```python
from build123d import *

# Parameters (mm, degrees)
SKETCH1_R           = 2
BOSS_EXTRUDE1_DEPTH = 8


with BuildPart() as part:
    # Sketch1 → Boss-Extrude1 (new body)
    with BuildSketch(Plane.XY):
        Polygon((-111.736544033, -14.131727984), (-9.968599743, -14.131727984), (0, -14.131727984), (0, 18.131727984), (-10, 18.131727984), (-10, 10.368272016), (-111.736544033, 10.368272016), (-111.736544033, 18.131727984), (-140, 18.131727984), (-140, -14.131727984), align=None)
        with Locations((-134, 8.131727984)):
            Circle(SKETCH1_R, mode=Mode.SUBTRACT)
        with Locations((-117.736544033, 8.131727984)):
            Circle(SKETCH1_R, mode=Mode.SUBTRACT)
        with Locations((-134, -8.131727984)):
            Circle(SKETCH1_R, mode=Mode.SUBTRACT)
        with Locations((-117.736544033, -8.131727984)):
            Circle(SKETCH1_R, mode=Mode.SUBTRACT)
        Polygon((-111.736544033, -7.631727984), (-111.736544033, 5.368272016), (-10, 5.368272016), (-10, -5.631727984), (-23.736544033, -5.631727984), (-24.236544033, -7.631727984), (-24.736544033, -7.631727984), (-25.236544033, -7.631727984), (-25.736544033, -5.631727984), (-26.736544033, -5.631727984), (-27.236544033, -7.631727984), (-27.736544033, -7.631727984), (-28.236544033, -7.631727984), (-28.736544033, -5.631727984), (-29.736544033, -5.631727984), (-30.236544033, -7.631727984), (-30.736544033, -7.631727984), (-31.236544033, -7.631727984), (-31.736544033, -5.631727984), (-32.736544033, -5.631727984), (-33.236544033, -7.631727984), (-33.736544033, -7.631727984), (-34.236544033, -7.631727984), (-34.736544033, -5.631727984), (-35.736544033, -5.631727984), (-36.236544033, -7.631727984), (-36.736544033, -7.631727984), (-37.236544033, -7.631727984), (-37.736544033, -5.631727984), (-38.736544033, -5.631727984), (-39.236544033, -7.631727984), (-39.736544033, -7.631727984), (-40.236544033, -7.631727984), (-40.736544033, -5.631727984), (-41.736544033, -5.631727984), (-42.236544033, -7.631727984), (-42.736544033, -7.631727984), (-43.236544033, -7.631727984), (-43.736544033, -5.631727984), (-44.736544033, -5.631727984), (-45.236544033, -7.631727984), (-45.736544033, -7.631727984), (-46.236544033, -7.631727984), (-46.736544033, -5.631727984), (-47.736544033, -5.631727984), (-48.236544033, -7.631727984), (-48.736544033, -7.631727984), (-49.236544033, -7.631727984), (-49.736544033, -5.631727984), (-50.736544033, -5.631727984), (-51.236544033, -7.631727984), (-51.736544033, -7.631727984), (-52.236544033, -7.631727984), (-52.736544033, -5.631727984), (-53.736544033, -5.631727984), (-54.236544033, -7.631727984), (-54.736544033, -7.631727984), (-55.236544033, -7.631727984), (-55.736544033, -5.631727984), (-56.736544033, -5.631727984), (-57.236544033, -7.631727984), (-57.736544033, -7.631727984), (-58.236544033, -7.631727984), (-58.736544033, -5.631727984), (-59.736544033, -5.631727984), (-60.236544033, -7.631727984), (-60.736544033, -7.631727984), (-61.236544033, -7.631727984), (-61.736544033, -5.631727984), (-62.736544033, -5.631727984), (-63.236544033, -7.631727984), (-63.736544033, -7.631727984), (-64.236544033, -7.631727984), (-64.736544033, -5.631727984), (-65.736544033, -5.631727984), (-66.236544033, -7.631727984), (-66.736544033, -7.631727984), (-67.236544033, -7.631727984), (-67.736544033, -5.631727984), (-68.736544033, -5.631727984), (-69.236544033, -7.631727984), (-69.736544033, -7.631727984), (-70.236544033, -7.631727984), (-70.736544033, -5.631727984), (-71.736544033, -5.631727984), (-72.236544033, -7.631727984), (-72.736544033, -7.631727984), (-73.236544033, -7.631727984), (-73.736544033, -5.631727984), (-74.736544033, -5.631727984), (-75.236544033, -7.631727984), (-75.736544033, -7.631727984), (-76.236544033, -7.631727984), (-76.736544033, -5.631727984), (-77.736544033, -5.631727984), (-78.236544033, -7.631727984), (-78.736544033, -7.631727984), (-79.236544033, -7.631727984), (-79.736544033, -5.631727984), (-80.736544033, -5.631727984), (-81.236544033, -7.631727984), (-81.736544033, -7.631727984), (-82.236544033, -7.631727984), (-82.736544033, -5.631727984), (-83.736544033, -5.631727984), (-84.236544033, -7.631727984), (-84.736544033, -7.631727984), (-85.236544033, -7.631727984), (-85.736544033, -5.631727984), (-86.736544033, -5.631727984), (-87.236544033, -7.631727984), (-87.736544033, -7.631727984), (-88.236544033, -7.631727984), (-88.736544033, -5.631727984), (-89.736544033, -5.631727984), (-90.236544033, -7.631727984), (-90.736544033, -7.631727984), (-91.236544033, -7.631727984), (-91.736544033, -5.631727984), (-92.736544033, -5.631727984), (-93.236544033, -7.631727984), (-93.736544033, -7.631727984), (-94.236544033, -7.631727984), (-94.736544033, -5.631727984), (-95.736544033, -5.631727984), (-96.236544033, -7.631727984), (-96.736544033, -7.631727984), (-97.236544033, -7.631727984), (-97.736544033, -5.631727984), (-98.736544033, -5.631727984), (-99.236544033, -7.631727984), (-99.736544033, -7.631727984), (-100.236544033, -7.631727984), (-100.736544033, -5.631727984), (-101.736544033, -5.631727984), (-102.236544033, -7.631727984), (-102.736544033, -7.631727984), (-103.236544033, -7.631727984), (-103.736544033, -5.631727984), (-104.736544033, -5.631727984), (-105.236544033, -7.631727984), (-105.736544033, -7.631727984), (-106.236544033, -7.631727984), (-106.736544033, -5.631727984), (-107.736544033, -5.631727984), (-108.236544033, -7.631727984), (-108.736544033, -7.631727984), (-109.236544033, -7.631727984), (-109.736544033, -5.631727984), (-110.736544033, -5.631727984), (-111.236544033, -7.631727984), align=None, mode=Mode.SUBTRACT)
    extrude(amount=BOSS_EXTRUDE1_DEPTH)


solid = part.part
```
Build history of the part. All positions in model axes, mm. A direction names the side the tool comes from. Give positions to 0.01 mm unless a question says otherwise; leave off trailing zeros. Loops run counter-clockwise (first coordinate to the right, second up) from the corner with the lowest first, then second, coordinate; pieces in that order, holes last.
Item 1: Slice it at C-C, the plane z = 5.5. Give the number of separate pieces and of enclosed holes in the cut face, and give its area (3 significant figures).
Answers follow:
separate pieces: 1
enclosed holes: 5
area: 2,470 mm2
Item 2: Slice it at B-B, the plane x = -134. List the corners of the cut face in (y, z), and give its area (3 significant figures).
Answers follow:
outline: (-14.13, 0) - (-10.13, 0) - (-10.13, 8) - (-14.13, 8) - close; (-6.13, 0) - (6.13, 0) - (6.13, 8) - (-6.13, 8) - close; (10.13, 0) - (18.13, 0) - (18.13, 8) - (10.13, 8) - close
area: 194 mm2
Item 3: Drill centre lines: line 1 (Y direction, x = -134, z = 6); line 2 (X direction, y = -8, z = 7); line 3 (X direction, y = 11, z = 0.75). Where is each one in solid material? Low to high.
Answers follow:
line 1: y = -14.13 to -10.13, -6.13 to 6.13, 10.13 to 18.13
line 2: x = -140 to -136, -132 to -119.73, -115.74 to 0
line 3: x = -140 to -111.74, -10 to 0
Item 4: Which spindle directions (+Z, -Z, +X, -X, +Y, -Y) get a long thin tool onto all of the face, cutting with end or side? Do faces 5 (the face through (-10, 0, 4)), 6 (the face through (-71, 6, 8)), 7 (the face through (-60, 10.368, 4)). Say none if no direction does.
Answers follow:
face 5: +Z, -Z
face 6: +Z, +X, -X, +Y, -Y
face 7: +Z, -Z, +Y
Item 5: Flat gauge pin, fed straight in: pin 1 (0.8 mm diameter, centred on x = -96.5, z = 3, fed in from +Y). Where does the tip first touch, or does it go through?
Answers follow:
pin 1: stops at y = 10.37
Item 6: Slice it at A-A, the plane y = 4. List the corners of the cut face in (x, z), and give its area (3 significant figures).
Answers follow:
outline: (-140, 0) - (-111.74, 0) - (-111.74, 8) - (-140, 8) - close; (-10, 0) - (0, 0) - (0, 8) - (-10, 8) - close
area: 306 mm2
Item 7: Pull direction X, two halves, no side cores. Call faces 1 (the face through (-140, 2, 4)), 2 (the face through (-119.735, 8.22, 3.944)), 3 (the face through (0, 2, 4)), 4 (the face through (-126, 18.132, 4)): released by +X, released by -X, zero draft, split by the parting line, or undercut.
Answers follow:
face 1: released by -X
face 2: undercut
face 3: released by +X
face 4: zero draft
